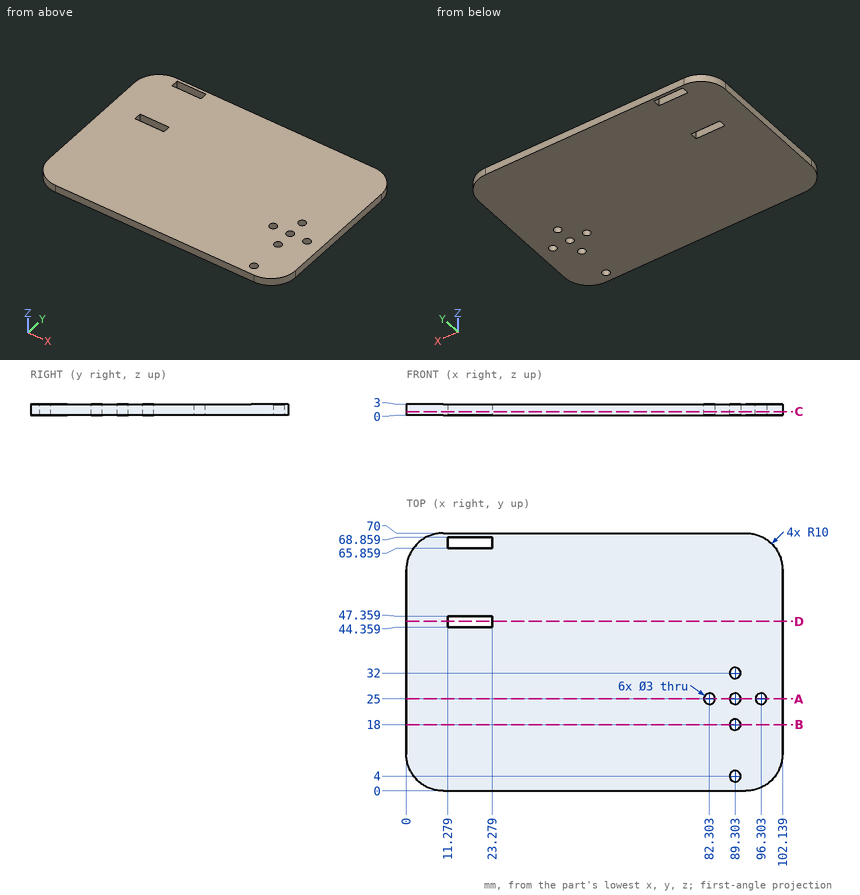
Study the drawing (mm; zero at the part's minimum x, y, z) and answer. Round coordinates to 2 decimals unless told otherwise and drop trailing zeros. Write each loop counter-clockwise with the first axis right and the second up, starting at its lowest first coordinate (ties: lowest second). Pieces come first, ordered by that corner, then holes. Notation, with made-up numbers: (4.5, 2) - (14.5, 2) arc R17 cw to (14.5, 14) - close; hole circle Ø4 at (1, -29). An arc over 180 degrees is marked (long way). Use a Markdown table: item, result. Add a question column.
1. The part is cut by section B-B (y = 18). Write down the section's boundary in (x, z).
2. The part is cut by section A-A (y = 25). Write down the section's boundary in (x, z).
3. The part is cut by section C-C (z = 0.95). Give the number of separate pieces and of enclosed holes in the cut face, and give its area (3 significant figures).
4. The part is cut by section D-D (y = 46). Write down the section's boundary in (x, z).
5. Consider line 1 (Y direction, x = 11.5, z = 2.75); line 2 (X direction, y = 32.5, z = 2.15); line 3 (X direction, y = 26, z = 2.8) (1 decimal). Determine where each line is inside the solid, lowest interval first.
Reported:
| question | item | result |
|---|---|---|
| 1 | outline | (0, 0) - (87.8, 0) - (87.8, 3) - (0, 3) - close; (90.8, 0) - (102.14, 0) - (102.14, 3) - (90.8, 3) - close |
| 2 | outline | (0, 0) - (80.8, 0) - (80.8, 3) - (0, 3) - close; (83.8, 0) - (87.8, 0) - (87.8, 3) - (83.8, 3) - close; (90.8, 0) - (94.8, 0) - (94.8, 3) - (90.8, 3) - close; (97.8, 0) - (102.14, 0) - (102.14, 3) - (97.8, 3) - close |
| 3 | separate pieces | 1 |
| 3 | enclosed holes | 8 |
| 3 | area | 6,950 mm^2 |
| 4 | outline | (0, 0) - (11.28, 0) - (11.28, 3) - (0, 3) - close; (23.28, 0) - (102.14, 0) - (102.14, 3) - (23.28, 3) - close |
| 5 | line 1 | 0 to 44.36, 47.36 to 65.86, 68.86 to 70 |
| 5 | line 2 | 0 to 87.89, 90.72 to 102.14 |
| 5 | line 3 | 0 to 81.2, 83.4 to 88.2, 90.4 to 95.2, 97.4 to 102.1 |
